Input: part model. Units: mm. Frame: model coordinates. A direction names the side the tool comes from. Give positions to 0.01 mm unless a question says otherwise; leave off trailing zeros. Write each loop counter-clockwise with the first axis right and the second up, starting at its lowest first coordinate (ties: lowest second). Pieces come first, ordered by that corner, then holes. Notation, with made-up numbers: (52.25, -7) - (58.25, -7) arc R18 cw to (58.25, 26) - close; hole circle Ø1 at (-28.75, 62). An arc over 180 degrees is marked (long way). Answer as CSV lines item,"result".
```python
from build123d import *

# Parameters (mm, degrees)
F0_W     = 127
F0_H     = 76.2
F1_DEPTH = 25.4
F2_R     = 19.05
F3_T     = -2.54
F4_R     = 6.35
F5_DEPTH = 22.86


with BuildPart() as f1:
    # F0 (on Right) → F1 (new body)
    with BuildSketch(Plane.YZ):
        with Locations((-63.5, 38.1)):
            Rectangle(F0_W, F0_H)
    extrude(amount=-F1_DEPTH)

    # F2
    f2_edges = [f1.edges().sort_by_distance(p)[0] for p in [
        (-12.7, -127, 76.2),
        (-12.7, -127, 0),
        (-12.7, 0, 76.2),
        (-12.7, 0, 0),
    ]]
    fillet(f2_edges, radius=F2_R)

    # F3
    f3_openings = [f1.faces().sort_by_distance(p)[0] for p in [
        (0, -63.5, 38.1),
    ]]
    offset(amount=F3_T, openings=f3_openings)

    # F4 (on face) → F5 (join, through all)
    with BuildSketch(Plane.YZ.offset(-22.86)):
        with Locations((-107.95, 57.15)):
            Circle(F4_R)
        with Locations((-107.95, 19.05)):
            Circle(F4_R)
    extrude(amount=F5_DEPTH)


solid = f1.part
```
Item 1: Contact query for flat-ended pins moving along their axis: pin 1 (1.5 mm diameter, centred on x = -10.5, z = 12.5, fed in from -Y); pin 2 (6 mm diameter, centred on x = -21, y = -13.5, fed in from +Z). Output: stop coordinate, or through.
The answers:
pin 1,"y = -126.1"
pin 2,"z = 76.03"
Item 2: Cut plane B-B on z = 37.5. Return the cut outline in (x, y).
The answers:
outline,"(-25.4, -127) - (0, -127) - (0, -124.46) - (-22.86, -124.46) - (-22.86, -2.54) - (0, -2.54) - (0, 0) - (-25.4, 0) - close"
Item 3: Cut plane A-A on x = -17.5. Return the cut outline in (y, z), plus the area to 3 significant figures.
The answers:
outline,"(-127, 19.05) arc R19.05 ccw to (-107.95, 0) - (-19.05, 0) arc R19.05 ccw to (0, 19.05) - (0, 57.15) arc R19.05 ccw to (-19.05, 76.2) - (-107.95, 76.2) arc R19.05 ccw to (-127, 57.15) - close; circle Ø12.7 at (-107.95, 19.05); circle Ø12.7 at (-107.95, 57.15); hole (-124.46, 19.05) arc R16.51 ccw to (-107.95, 2.54) - (-19.05, 2.54) arc R16.51 ccw to (-2.54, 19.05) - (-2.54, 57.15) arc R16.51 ccw to (-19.05, 73.66) - (-107.95, 73.66) arc R16.51 ccw to (-124.46, 57.15) - close"
area,"1,180 mm²"
Item 4: Cut plane C-C on y = -23.5. Return the cut outline in (x, z), plus the area to 3 significant figures.
The answers:
outline,"(-25.4, 0) - (0, 0) - (0, 2.54) - (-22.86, 2.54) - (-22.86, 73.66) - (0, 73.66) - (0, 76.2) - (-25.4, 76.2) - close"
area,"310 mm²"
Item 5: Ray query, line 1 (Y direction, x = -15.5, z = 57); line 2 (Y direction, x = -1.5, z = 45); line 3 (Z direction, x = -9.75, y = -59.5). Return the intervals inside material, ascending. Write a range as from..to.
The answers:
line 1,"-127..-124.46, -114.3..-101.6, -2.54..0"
line 2,"-127..-124.46, -2.54..0"
line 3,"0..2.54, 73.66..76.2"
Item 6: Cut plane D-D on z = 16. Return the cut outline in (x, y), plus the area to 3 significant figures.
The answers:
outline,"(-25.4, -126.75) - (0, -126.75) - (0, -124.18) - (-22.86, -124.18) - (-22.86, -113.52) - (0, -113.52) - (0, -102.38) - (-22.86, -102.38) - (-22.86, -2.82) - (0, -2.82) - (0, -0.25) - (-25.4, -0.25) - close"
area,"694 mm²"
Item 7: Mould query, pull axis Z, two halves, no side actions, for faces 3 (the face through (-12.88, -5.73, 5.43)), 4 (the face through (-11, -64, 2.54)), 5 (the face through (-13, -127, 38)). Classes: +Z half, -Z half, draft (parallel to the pull), parting line (faces both ways), or undercut.
The answers:
face 3,"-Z half"
face 4,"undercut"
face 5,"draft"
Item 8: Reachability of faces 1 (the face through (-11, -124.46, 38)), 2 (the face through (0, -108, 19)) from +Z, -Z, +X, -X, +Y, -Y: full face, straight path, thin tool, end or side. Return the list, or none.
The answers:
face 1,"+X"
face 2,"+Z, -Z, +X, +Y, -Y"
